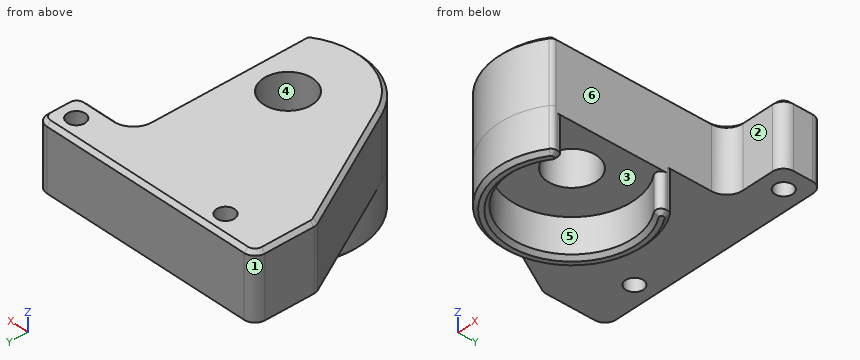
```python
from build123d import *

# Parameters (mm, degrees)
SKETCH027_R     = 1.65
SKETCH027_R_2   = 4.5
PAD014_DEPTH    = 12
SKETCH028_R     = 4.5
PAD015_DEPTH    = 8
SKETCH029_R     = 11.25
POCKET006_DEPTH = 7
FILLET001_R     = 3
FILLET003_R     = 1
FILLET004_R     = 2
CHAMFER010_SIZE = 0.7


with BuildPart() as part:
    # Sketch027 → Pad014 (new body)
    with BuildSketch(Plane.XY):
        with BuildLine():
            ThreePointArc((-11.900838, -6.373387), (-2.978027, -13.167435), (8, -10.874282))
            Line((8, -10.874282), (8, 21.5))
            Line((8, 21.5), (19, 21.5))
            Line((19, 21.5), (19, 29))
            Line((19, 29), (-24.657124, 29))
            Line((-24.657124, 29), (-24.657124, 17.446049))
            Line((-24.657124, 17.446049), (-11.900838, -6.373387))
        make_face()
        with Locations((15, 25.4)):
            Circle(SKETCH027_R, mode=Mode.SUBTRACT)
        with Locations((-15, 25.4)):
            Circle(SKETCH027_R, mode=Mode.SUBTRACT)
        Circle(SKETCH027_R_2, mode=Mode.SUBTRACT)
    extrude(amount=PAD014_DEPTH)

    # Sketch028 (on Face11 of Pad014) → Pad015 (join)
    with BuildSketch(Plane(origin=(0, 0, 0), x_dir=(1, 0, 0), z_dir=(0, 0, -1))):
        with BuildLine():
            ThreePointArc((8, 10.874282), (-13.5, 0), (8, -10.874282))
            Line((8, -10.874282), (8, 10.874282))
        make_face()
        Circle(SKETCH028_R, mode=Mode.SUBTRACT)
    extrude(amount=PAD015_DEPTH)

    # Sketch029 (on Face1 of Pad015) → Pocket006 (cut)
    with BuildSketch(Plane(origin=(0, 0, -8), x_dir=(1, 0, 0), z_dir=(0, 0, -1))):
        Circle(SKETCH029_R)
    extrude(amount=-POCKET006_DEPTH, mode=Mode.SUBTRACT)

    # Fillet001
    fillet001_edges = [part.edges().sort_by_distance(p)[0] for p in [
        (8, 21.5, 6),
    ]]
    fillet(fillet001_edges, radius=FILLET001_R)

    # Fillet003
    fillet003_edges = [part.edges().sort_by_distance(p)[0] for p in [
        (8, -10.874282, 2),
        (8, -7.909646, -4.5),
        (8, 7.909646, -4.5),
        (8, 10.874282, -4),
    ]]
    fillet(fillet003_edges, radius=FILLET003_R)

    # Fillet004
    fillet004_edges = [part.edges().sort_by_distance(p)[0] for p in [
        (19, 21.5, 6),
        (19, 29, 6),
        (-24.657124, 17.446049, 6),
        (-24.657124, 29, 6),
    ]]
    fillet(fillet004_edges, radius=FILLET004_R)

    # Chamfer010
    chamfer010_edges = [part.edges().sort_by_distance(p)[0] for p in [
        (-24.657124, 22.473937, 12),
        (-13.5, 0, -8),
    ]]
    chamfer(chamfer010_edges, length=CHAMFER010_SIZE)


with BuildPart() as part_1:
    # Body012 placement: moved
    add(part.part.moved(Location((0, -32, 50))))


solid = part_1.part
```
For this review, take the finished solid that the model builds, in its own axes (mm). Face numbers are marked on the shaded views. A direction names the side the tool comes from. Coordinates: 2 decimals unless noted, no trailing zeros. Write each loop counter-clockwise with the first axis right and the second up, starting at its lowest first coordinate (ties: lowest second). Pieces come first, ordered by that corner, then holes. Notation, with made-up numbers: (-27, 70.5) - (9, 70.5) arc R25 cw to (9, 89.5) - close; hole circle Ø6 at (19, 22). An arc over 180 degrees is marked (long way). Put each result on its own line as item: value.
1. Add section D-D, the plane y = -32. Give the boundary of the cut face in (x, z).
Values found:
outline: (-15.31, 50) - (-13.5, 50) - (-13.5, 42.7) - (-12.8, 42) - (-11.95, 42) - (-11.25, 42.7) - (-11.25, 49) - (-4.5, 49) - (-4.5, 62) - (-14.52, 62) - (-15.31, 61.3) - close; (4.5, 49) - (8, 49) - (8, 61.3) - (7.3, 62) - (4.5, 62) - close
2. Mouldability with a two-part tool opening along X and no side actions: class the marked faces 1, 2 and 3 as released by +X, released by -X, zero draft, split by the parting line, or undercut.
Values found:
face 1: released by -X
face 2: zero draft
face 3: undercut
3. Add section B-B, the plane x = 15. Give the boundary of the cut face in (y, z).
Values found:
outline: (-10.5, 50) - (-8.25, 50) - (-8.25, 62) - (-9.8, 62) - (-10.5, 61.3) - close; (-4.95, 50) - (-3, 50) - (-3, 61.3) - (-3.7, 62) - (-4.95, 62) - close
4. Add section A-A, the plane z = 55.75. Give the boundary of the cut face in (x, y), then the cut area to 3 significant figures.
Values found:
outline: (-24.66, -14.05) arc R2 ccw to (-24.42, -15) - (-11.9, -38.37) arc R13.5 ccw to (7.56, -43.18) arc R1 ccw to (8, -42.36) - (8, -13.5) arc R3 cw to (11, -10.5) - (17, -10.5) arc R2 ccw to (19, -8.5) - (19, -5) arc R2 ccw to (17, -3) - (-22.66, -3) arc R2 ccw to (-24.66, -5) - close; hole circle Ø3.3 at (-15, -6.6); hole circle Ø9 at (0, -32); hole circle Ø3.3 at (15, -6.6)
area: 1,120 mm²
5. Wall thickness on probe 1 along X at (y, z) = (-7, 58.5); probe 2 along Y at (x, z) = (15, 57.25); probe 3 along Z at (x, y) = (-1.5, -42.5): over which ranges is each line inside the solid? List them lowest first.
Values found:
probe 1: -24.66 to -16.6, -13.4 to 13.4, 16.6 to 19
probe 2: -10.5 to -8.25, -4.95 to -3
probe 3: 49 to 62
6. For pin 1 (13.5 mm diameter, centred on x = 0, y = -32, fed in from -Z); pin 2 (1 mm diameter, centred on y = -32.5, z = 50.5, fed in from -X); pin 3 (9.5 mm diameter, centred on y = -30.5, z = 56.5, fed in from +X); pin 4 (5 mm diameter, centred on y = -8.5, z = 47, fed in from +X), all flat-tipped, find the tip position at first contact; note any pin that passes through.
Values found:
pin 1: z = 49
pin 2: x = -15.31
pin 3: x = 8
pin 4: through
7. Machinability: for the marked faces 4, 5 and 6, which of the approach directions +Z, -Z, +X, -X, +Y, -Y give a long, thin tool a straight path to every point of the face, cutting with its end or side? Answer none if there is none.
Values found:
face 4: +Z, -Z
face 5: -Z
face 6: +Z, -Z, +X, -Y
8. Add section C-C, the plane y = -6.6. Give the boundary of the cut face in (x, z).
Values found:
outline: (-24.66, 50) - (-16.65, 50) - (-16.65, 62) - (-23.96, 62) - (-24.66, 61.3) - close; (-13.35, 50) - (13.35, 50) - (13.35, 62) - (-13.35, 62) - close; (16.65, 50) - (19, 50) - (19, 61.3) - (18.3, 62) - (16.65, 62) - close
